For this review, take the finished solid that the model builds, in its own axes (mm). A direction names the side the tool comes from. Give positions to 0.01 mm unless a question says otherwise; leave off trailing zeros. Order: outer loops, then holes, each group sorted by start corner. A loop starts at its lowest first (then second) coordinate and runs counter-clockwise, first axis right, second up. Notation, with made-up numbers: (36, -10.5) - (62, -10.5) arc R26 cw to (62, 25.5) - close; hole circle Ø8 at (24.25, -31.75). An arc over 180 degrees is marked (long way). One line per item, written item: value.
Autodesk Inventor part; units mm, degrees
ref_plane "YZ Plane" through (0, 0, 0) normal (1, 0, 0) x (0, 1, 0)
ref_plane "XZ Plane" through (0, 0, 0) normal (0, 1, 0) x (-1, 0, 0)
ref_plane "XY Plane" through (0, 0, 0) normal (0, 0, 1) x (1, 0, 0)
sketch "Sketch1" plane through (0, 0, 0) normal (0, 1, 0) x (-1, 0, 0)
  line L0 (0, 0) -> (40.8, 0)
  line L1 (40.8, 0) -> (40.8, -40.25)
  line L2 (40.8, -40.25) -> (0, -40.25)
  line L3 (0, -40.25) -> (0, 0)
  dimension "d0" = 40.8
  dimension "d1" = 40.25
extrude "Extrusion1" add sketch "Sketch1" along normal blind 20.35
sketch "Sketch2" plane through (0, 20.35, 0) normal (0, 1, 0) x (1, 0, 0)
  line L0 (-40.8, 0) -> (0, 0)
  line L1 (-40.8, 0) -> (-40.8, 4.68)
  line L2 (-40.8, 40.25) -> (-40.8, 0)
  line L3 (-40.8, 0) -> (-37.8, 0)
  line L4 (-37.8, 0) -> (-38.396, 2.1177)
  line L5 (-38.396, 2.1177) -> (-40.8, 4.68)
  dimension "d4" = 4.68
  dimension "d5" = 3
  dimension "d6" = 2.2
extrude "Extrusion2" cut sketch "Sketch2" against normal blind 20.35
sketch "Sketch3" plane through (0, 20.35, 0) normal (0, 1, 0) x (1, 0, 0)
  line L0 (-40.8, 4.68) -> (-40.8, 40.25)
  line L1 (-40.8, 40.25) -> (-36.8, 40.25)
  line L2 (-40.8, 40.25) -> (0, 40.25)
  line L3 (-40.8, 40.25) -> (-40.8, 35.25)
  line L4 (-40.8, 35.25) -> (-36.8, 40.25)
  point P0 (0, 0)
  dimension "d9" = 4
  dimension "d10" = 5
extrude "Extrusion3" cut sketch "Sketch3" against normal blind 20.35
sketch "Sketch4" plane through (-40.8, 0, -4.68) normal (-1, 0, 0) x (0, 0, 1)
  circle A0 centre (-25.57, 10.175) radius 2.625
  line L0 (-35.57, 0) -> (-35.57, 20.35)
  line L1 (-30.57, 20.35) -> (0, 20.35)
  point P0 (4.68, 0)
  dimension "d13" = 5.25
  dimension "d14" = 10
  dimension "d15" = 10.175
extrude "Extrusion4" add sketch "Sketch4" along normal blind 1.5
sketch "Sketch5" plane through (-42.3, 10.175, -30.25) normal (-1, 0, 0) x (0, 0, 1)
  circle A0 centre (0, 0) radius 4.375
  point P0 (30.25, -10.175)
  dimension "d18" = 8.75
extrude "Extrusion5" add sketch "Sketch5" along normal blind 2.8
sketch "Sketch6" plane through (-45.1, 10.175, -30.25) normal (-1, 0, 0) x (0, 0, 1)
  circle A0 centre (0, 0) radius 10
  point P0 (30.25, -10.175)
  dimension "d21" = 20
extrude "Extrusion6" add sketch "Sketch6" along normal blind 2.2
sketch "Sketch7" plane through (0, 0, 0) normal (0, 0, 1) x (1, 0, 0)
  line L0 (-7, 6.875) -> (-3.25, 6.875)
  line L1 (-3.25, 6.875) -> (-3.25, 13.475)
  line L2 (-3.25, 13.475) -> (-7, 13.475)
  line L3 (-7, 13.475) -> (-7, 6.875)
  line L4 (0, 0) -> (0, 20.35)
  line L5 (0, 0) -> (-37.8, 0)
  dimension "d24" = 3.75
  dimension "d25" = 6.6
  dimension "d26" = 7
  dimension "d27" = 6.875
extrude "Extrusion7" add sketch "Sketch7" along normal blind 4.5
chamfer "Chamfer1" distance 2 angle 45 2 edges at (-5.125, 13.475, 4.5) (-5.125, 6.875, 4.5)
sketch "Sketch8" plane through (-7, 6.875, 0) normal (-1, 0, 0) x (0, 0, 1)
  line L0 (0, 6.6) -> (0, 0)
  line L1 (0, 0) -> (0, 6.6)
  line L2 (0, 6.6) -> (2.5, 6.6)
  line L3 (0, 6.6) -> (2.5, 6.6)
  line L4 (4.5, 4.6) -> (4.5, 2)
  line L5 (2.5, 6.6) -> (4.5, 4.6)
  line L6 (4.5, 4.6) -> (4.5, 2)
  line L7 (4.5, 2) -> (2.5, 0)
  line L8 (4.5, 2) -> (2.5, 0)
  line L9 (0, 0) -> (2.5, 0)
  line L10 (2.5, 0) -> (0, 0)
  point P0 (0, -6.875)
extrude "Extrusion8" cut sketch "Sketch8" against normal blind 4.5
sketch "Sketch9" plane through (0, 0, -40.25) normal (0, 0, -1) x (-1, 0, 0)
  line L0 (3.25, 6.875) -> (7, 6.875)
  line L1 (7, 6.875) -> (7, 13.475)
  line L2 (7, 13.475) -> (3.25, 13.475)
  line L3 (3.25, 13.475) -> (3.25, 6.875)
  line L4 (0, 20.35) -> (36.8, 20.35)
  line L5 (0, 0) -> (0, 20.35)
  dimension "d35" = 3.75
  dimension "d36" = 6.6
  dimension "d37" = 6.875
  dimension "d45" = 7
extrude "Extrusion9" add sketch "Sketch9" along normal blind 4.5
chamfer "Chamfer2" distance 1 angle 45 2 edges at (-5.125, 6.875, -44.75) (-5.125, 13.475, -44.75)
sketch "Sketch10" plane through (-7, 6.875, -40.25) normal (-1, 0, 0) x (0, 0, 1)
  line L0 (0, 0) -> (0, 6.6)
  line L1 (-4.5, 1) -> (-4.5, 5.6)
  line L2 (0, 0) -> (-4.5, 1)
  line L3 (0, 0) -> (-3.5, 0)
  line L4 (-4.5, 1) -> (-3.5, 0)
  line L5 (-3.5, 0) -> (0, 0)
  line L6 (0, 6.6) -> (-3.5, 6.6)
  line L7 (-4.5, 5.6) -> (-3.5, 6.6)
  line L8 (-3.5, 6.6) -> (0, 6.6)
  line L9 (0, 6.6) -> (-4.5, 5.6)
  point P0 (40.25, -6.875)
extrude "Extrusion10" cut sketch "Sketch10" against normal blind 4.5 contours L3 L4 L2 | L9 L7 L6
sketch "Sketch11" plane through (0, 0, -40.25) normal (0, 0, -1) x (-1, 0, 0)
  line L0 (0, 20.35) -> (36.8, 20.35)
  line L1 (27, 0) -> (30, 0)
  line L2 (30, 0) -> (30, 20.35)
  line L3 (30, 20.35) -> (27, 20.35)
  line L4 (27, 20.35) -> (27, 0)
  line L5 (0, 0) -> (0, 20.35)
  dimension "d46" = 3
  dimension "d47" = 27
extrude "Extrusion11" add sketch "Sketch11" along normal blind 1.5
sketch "Sketch12" plane through (0, 0, 0) normal (0, 0, 1) x (1, 0, 0)
  line L0 (0, 0) -> (-37.8, 0)
  line L1 (0, 20.35) -> (-27, 20.35)
  line L2 (-27, 0) -> (-30, 0)
  line L3 (-30, 0) -> (-30, 20.35)
  line L4 (-30, 20.35) -> (-27, 20.35)
  line L5 (-27, 20.35) -> (-27, 0)
  line L6 (0, 0) -> (0, 20.35)
  dimension "d50" = 3
  dimension "d51" = 27
extrude "Extrusion12" add sketch "Sketch12" along normal blind 1.5 contours L0 L3 L4 L5
properties part number "DS3218_motor"
(1) Take a section at A-A (y = 2.25). Write out the cut boundary in (x, z), then the cut area to 3 significant figures.
Answers below:
outline: (-47.3, -36.35) - (-45.1, -36.35) - (-45.1, -24.15) - (-47.3, -24.15) - close; (-40.8, -35.25) - (-36.8, -40.25) - (-30, -40.25) - (-30, -41.75) - (-27, -41.75) - (-27, -40.25) - (0, -40.25) - (0, 0) - (-27, 0) - (-27, 1.5) - (-30, 1.5) - (-30, 0) - (-37.8, 0) - (-38.4, -2.12) - (-40.8, -4.68) - close
area: 1,660 mm^2
(2) Take a section at B-B (z = -39). Write out the cut boundary in (x, y).
Answers below:
outline: (-47.3, 5.33) - (-45.1, 5.33) - (-45.1, 15.02) - (-47.3, 15.02) - close; (-37.8, 0) - (0, 0) - (0, 20.35) - (-37.8, 20.35) - close
(3) Take a section at D-D (z = -21). Write out the cut boundary in (x, y), then the cut area to 3 significant figures.
Answers below:
outline: (-47.3, 6.38) - (-45.1, 6.38) - (-45.1, 13.97) - (-47.3, 13.97) - close; (-40.8, 0) - (0, 0) - (0, 20.35) - (-40.8, 20.35) - close
area: 847 mm^2
(4) Machinability: for faces 1 (the face through (-34, 10, 0)), 2 (the face through (-13, 10, 0)), 3 (the face through (-33, 10, -40.25)), which of the approach directions +Z, -Z, +X, -X, +Y, -Y give a long, thin tool a straight path to every point of the face, cutting with its end or side? Answer none if there is none.
Answers below:
face 1: +Z, -X, +Y, -Y
face 2: +Z, +X, +Y, -Y
face 3: -Z, -X, +Y, -Y
(5) Draft analysis for pull direction X (two halves, no side actions). For faces 4 (the face through (-7, 10, -42)), 5 (the face through (-30, 10, -41)), 6 (the face through (-3.25, 10, -42)), state which applies: pulls with the +X half, pulls with the -X half, needs draft (parallel to the pull), parting line crosses it, or undercut.
Answers below:
face 4: undercut
face 5: pulls with the -X half
face 6: pulls with the +X half
(6) For P1, Ø3.5, axis at y = 11, z = -42.5, coming from the +X side; P2, Ø1.5, axis at y = 14.5, z = -6, coming from the -X side; P3, Ø4, axis at x = -35, y = 5, coming from the +Z side, all flat-tipped, find the tip position at first contact; note any pin that passes through.
Answers below:
P1: stops at x = -3.25
P2: stops at x = -40.8
P3: stops at z = 0
(7) Wall thickness on line 1 (X direction, y = 12.25, z = -27.5); line 2 (X direction, y = 17, z = -28); line 3 (X direction, y = 2.5, z = -9.5): over which ranges is each line inside the solid? List them lowest first. Write a range as from..to.
Answers below:
line 1: x = -47.3..-42.3, -40.8..0
line 2: x = -47.3..-45.1, -40.8..0
line 3: x = -40.8..0
(8) Take a section at C-C (z = -30.25). Write out the cut boundary in (x, y) (3 decimals), then the cut area to 3 significant figures.
Answers below:
outline: (-47.3, 0.175) - (-45.1, 0.175) - (-45.1, 5.8) - (-42.3, 5.8) - (-42.3, 7.55) - (-40.8, 7.55) - (-40.8, 0) - (0, 0) - (0, 20.35) - (-40.8, 20.35) - (-40.8, 12.8) - (-42.3, 12.8) - (-42.3, 14.55) - (-45.1, 14.55) - (-45.1, 20.175) - (-47.3, 20.175) - close
area: 907 mm^2
